Build history of the part. All positions in model axes, mm. Face numbers are marked on the shaded views. Round coordinates to 2 decimals unless told otherwise and drop trailing zeros. Write each loop counter-clockwise with the first axis right and the second up, starting at its lowest first coordinate (ties: lowest second). Pieces come first, ordered by that corner, then holes. Notation, with made-up numbers: M -33,31.5 L -23,31.5 A3 cw -23,36.5 Z; hole C 16.25,53.5 d10. An arc over 180 degrees is marked long. Write item = value, one per line.
from build123d import *

# Parameters (mm, degrees)
SKETCH_R          = 16.7005
SKETCH_R_2        = 13.3223
PAD_DEPTH         = 140
SKETCH001_W       = 20
SKETCH001_H       = 40
POCKET_DEPTH      = 16.7015
POCKET_DEPTH_BACK = -16.7015


with BuildPart() as part:
    # Sketch → Pad (new body)
    with BuildSketch(Plane.XY):
        Circle(SKETCH_R)
        Circle(SKETCH_R_2, mode=Mode.SUBTRACT)
    extrude(amount=PAD_DEPTH)

    # Sketch001 → Pocket (cut, two sides)
    with BuildSketch(Plane(origin=(0, 0, 140), x_dir=(1, 0, 0), z_dir=(0, -1, 0))) as pocket_sk:
        with Locations((0, -20)):
            Rectangle(SKETCH001_W, SKETCH001_H)
    extrude(amount=-POCKET_DEPTH, mode=Mode.SUBTRACT)
    extrude(pocket_sk.sketch, amount=-POCKET_DEPTH_BACK, mode=Mode.SUBTRACT)


solid = part.part
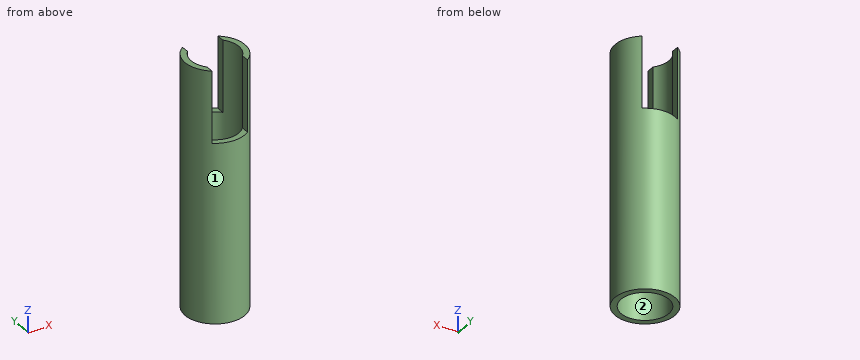
1. Band-saw the part on B-B (x = 0). List the corners of the cut face in (y, z), plus the area to 3 significant figures.
Responses:
outline = M -16.7,0 L -13.32,0 L -13.32,100 L -16.7,100 Z; M 13.32,0 L 16.7,0 L 16.7,100 L 13.32,100 Z
area = 676 mm²
2. Probe probe 1 along X at (y, z) = (0, 31); probe 2 along X at (y, z) = (10, 53). List the from-to ranges inside material, lowest first.
Responses:
probe_1 = -16.7 to -13.32, 13.32 to 16.7
probe_2 = -13.38 to -8.8, 8.8 to 13.38
3. Band-saw the part on A-A (y = -10). List the corners of the cut face in (x, z).
Responses:
outline = M -13.38,0 L -8.8,0 L -8.8,100 L -10,100 L -10,140 L -13.38,140 Z; M 8.8,0 L 13.38,0 L 13.38,140 L 10,140 L 10,100 L 8.8,100 Z
4. Mould opens along X. For the marked faces 1 and 2 say: pulls with the +X half, pulls with the -X half, needs draft (parallel to the pull), parting line crosses it, or undercut.
Responses:
face_1 = parting line crosses it
face_2 = undercut
5. Band-saw the part on D-D (z = 85). List the corners of the cut face in (x, y), plus the area to 3 significant figures.
Responses:
outline = C 0,0 d33.4; hole C 0,0 d26.64
area = 319 mm²
6. Band-saw the part on C-C (y = 0). List the corners of the cut face in (x, z).
Responses:
outline = M -16.7,0 L -13.32,0 L -13.32,140 L -16.7,140 Z; M 13.32,0 L 16.7,0 L 16.7,140 L 13.32,140 Z
7. Flat gauge pins, fed straight in: pin 1 (4 mm diameter, centred on x = 2, y = -13, fed in from +Z); pin 2 (8 mm diameter, centred on x = 3.5, z = 121, fed in from +Y); pin 3 (1.4 mm diameter, centred on y = -11.5, z = 112, fed in from +X); pin 4 (3.5 mm diameter, centred on y = -10.5, z = 111, fed in from -X). Where does each tip first touch, or does it go through?
Responses:
pin_1 = 100
pin_2 = through
pin_3 = 12.74
pin_4 = -14.22
